CAD build for the part. Positions are in the model's coordinates, mm. A direction names the side the tool comes from. Coordinates: 2 decimals unless noted, no trailing zeros. Order: outer loops, then holes, each group sorted by start corner. A loop starts at its lowest first (then second) coordinate and runs counter-clockwise, first axis right, second up. Notation, with made-up numbers: M 10,5.25 L 47,5.25 A14 cw 47,24.25 Z; hole C 88.5,-9.75 d9. An arc over 180 degrees is marked long. One line per item, written item: value.
from build123d import *

# Parameters (mm, degrees)
AUFSATZ_LINEAR_AUSTRAGEN1_DEPTH = 3
SKIZZE2_R                       = 2
AUFSATZ_LINEAR_AUSTRAGEN2_DEPTH = 17
AUFSATZ_LINEAR_START            = 15
AUFSATZ_LINEAR_AUSTRAGEN3_DEPTH = 1.6
SCHNITT_LINEAR_AUSTRAGEN1_REACH = 23.715
SKIZZE4_R                       = 1
FASE1_SIZE                      = 0.4


with BuildPart() as part:
    # Skizze1 → Aufsatz-Linear austragen1 (new body)
    with BuildSketch(Plane.XY):
        with BuildLine():
            Line((0, 2), (-5, 2))
            ThreePointArc((-5, 2), (-7, 0), (-5, -2))
            Line((-5, -2), (0, -2))
            ThreePointArc((0, -2), (2, 0), (0, 2))
        make_face()
    extrude(amount=AUFSATZ_LINEAR_AUSTRAGEN1_DEPTH)

    # Skizze2 → Aufsatz-Linear austragen2 (add)
    with BuildSketch(Plane.XY.offset(3)):
        with Locations(Location((0, 0, 0), (0, 0, 90))):
            Circle(SKIZZE2_R)
    extrude(amount=AUFSATZ_LINEAR_AUSTRAGEN2_DEPTH)

    # Skizze3 → Aufsatz-Linear austragen3 (add)
    with BuildSketch(Plane.XY.offset(3).offset(AUFSATZ_LINEAR_START)):
        with BuildLine():
            Line((-1.25, 3.5), (-1.25, 1.5612495))
            ThreePointArc((-1.25, 1.5612495), (0, 2), (1.25, 1.5612495))
            Line((1.25, 1.5612495), (1.25, 3.5))
            ThreePointArc((1.25, 3.5), (0, 4.75), (-1.25, 3.5))
        make_face()
    extrude(amount=AUFSATZ_LINEAR_AUSTRAGEN3_DEPTH)

    # Skizze4 → Schnitt-Linear austragen1 (cut, up to next)
    with BuildSketch(Plane.XY.offset(20), mode=Mode.PRIVATE) as schnitt_linear_austragen1_sk1:
        Circle(SKIZZE4_R)
    schnitt_linear_austragen1_tool1 = extrude(schnitt_linear_austragen1_sk1.sketch, amount=-SCHNITT_LINEAR_AUSTRAGEN1_REACH, mode=Mode.PRIVATE) & part.part
    add(schnitt_linear_austragen1_tool1.solids().sort_by_distance((0, 0, 20))[0], mode=Mode.SUBTRACT)

    # Fase1
    fase1_edges = [part.edges().sort_by_distance(p)[0] for p in [
        (0, -2, 20),
    ]]
    chamfer(fase1_edges, length=FASE1_SIZE - 0.0001)  # a hair under: the kernel refuses the full size


solid = part.part
Q1. Drill centre lines: line 1 along Y through (x, z) = (0, 11); line 2 along Z through (x, y) = (-1, 3); line 3 along Z through (x, y) = (-2, 0.5). Where is each one in solid material? Low to high.
Recorded:
line 1: y = -2 to -1, 1 to 2
line 2: z = 18 to 19.6
line 3: z = 0 to 3
Q2. Mould opens along X. For faces 3 (the face through (-1.25, 3, 19)), 4 (the face through (0, -1, 10)), 5 (the face through (-2, 2, 1)) say: released by +X, released by -X, zero draft, split by the parting line, or undercut.
Recorded:
face 3: released by -X
face 4: undercut
face 5: zero draft
Q3. Which spindle directions (+Z, -Z, +X, -X, +Y, -Y) get a long thin tool onto all of the face, cutting with end or side? Do faces 1 (the face through (1.25, 3, 19)), 2 (the face through (-3, -2, 1)). Say none if no direction does.
Recorded:
face 1: +Z, -Z, +X, +Y
face 2: +Z, -Z, +X, -X, -Y
Q4. Slice it at B-B (x = -3.75). List the corners of the cut face in (y, z).
Recorded:
outline: M -2,0 L 2,0 L 2,3 L -2,3 Z
Q5. Pin check, flat tips, straight feed: pin 1 Ø0.8 at (y, z) = (2.5, 19) entering from +X; pin 2 Ø2 at (y, z) = (1, 7.5) entering from -X; pin 3 Ø1.5 at (x, z) = (-1.5, 1) entering from +Y. Stop position of each tip, or through.
Recorded:
pin 1: stops at x = 1.25
pin 2: stops at x = -2
pin 3: stops at y = 2
Q6. Slice it at C-C (z = 11.25). List the corners of the cut face in (x, y).
Recorded:
outline: C 0,0 d4; hole C 0,0 d2
Q7. Slice it at D-D (x = -5.25). List the corners of the cut face in (y, z).
Recorded:
outline: M -1.98,0 L 1.98,0 L 1.98,3 L -1.98,3 Z
